Part print with two shaded views. Sizes in mm from the minimum x, y, z corner. A direction names the side the tool comes from. Give positions to 0.01 mm unless a question says otherwise; leave off trailing zeros. Order: outer loops, then holes, each group sorted by start corner. A loop starts at its lowest first (then second) coordinate and runs counter-clockwise, first axis right, second up. Notation, with made-up numbers: (-2.5, 0.25) -> (17.5, 0.25) arc R8 cw to (17.5, 12.25) -> close; hole circle Ø10 at (46, 16). An arc over 180 degrees is marked (long way). Answer as CSV lines item,"result".
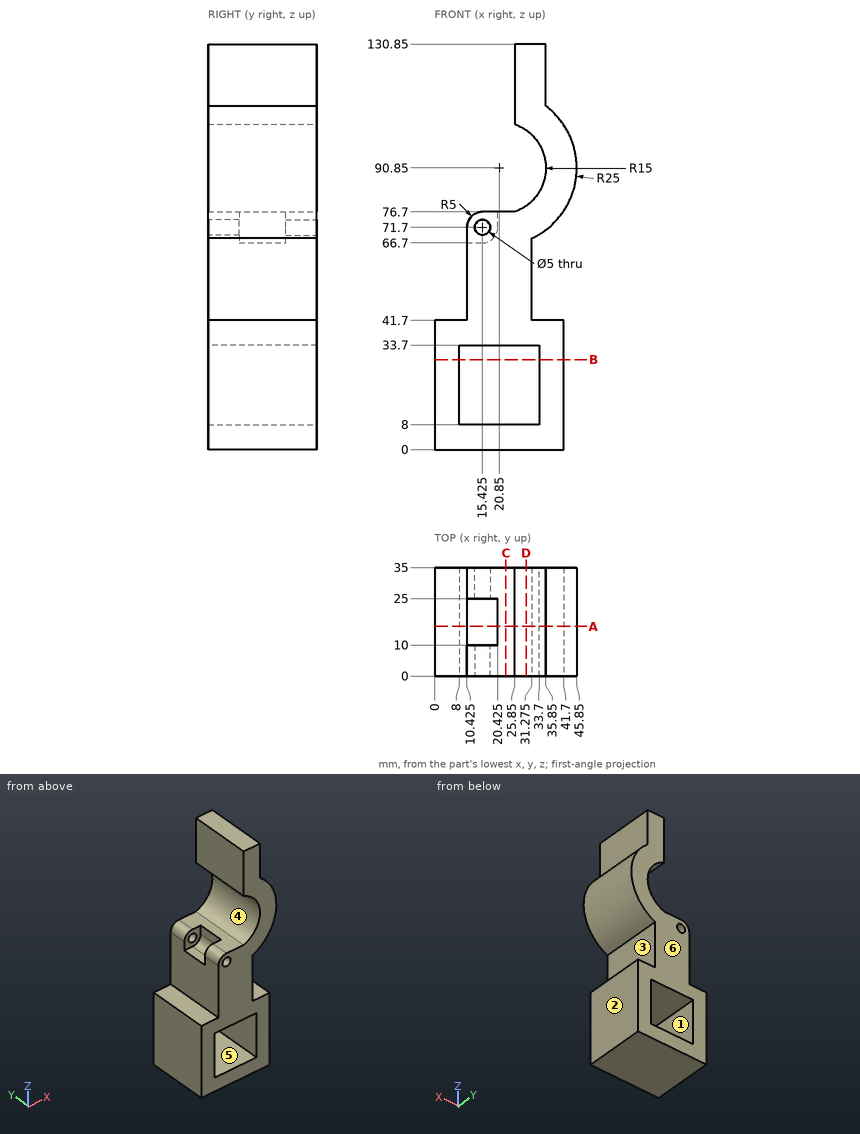
1) Band-saw the part on D-D, the plane x = 29.5. Write the cut outline in (y, z), then the cut area to 3 significant figures.
Data:
outline,"(0, 0) -> (35, 0) -> (35, 8) -> (0, 8) -> close; (0, 33.7) -> (35, 33.7) -> (35, 78.6) -> (0, 78.6) -> close; (0, 103.1) -> (35, 103.1) -> (35, 130.85) -> (0, 130.85) -> close"
area,"2,820 mm2"
2) Band-saw the part on A-A, the plane y = 16. Write the cut outline in (x, z) (3 decimals).
Data:
outline,"(0, 0) -> (41.7, 0) -> (41.7, 41.7) -> (31.275, 41.7) -> (31.275, 68.127) arc R25 ccw to (35.85, 110.85) -> (35.85, 130.85) -> (25.85, 130.85) -> (25.85, 104.992) arc R15 cw to (25.828, 76.7) -> (20.425, 76.7) -> (20.425, 71.7) arc R5 cw to (15.425, 66.7) -> (10.425, 66.7) -> (10.425, 41.7) -> (0, 41.7) -> close; hole (8, 8) -> (33.7, 8) -> (33.7, 33.7) -> (8, 33.7) -> close"
3) Band-saw the part on C-C, the plane x = 23. Write the cut outline in (y, z).
Data:
outline,"(0, 0) -> (35, 0) -> (35, 8) -> (0, 8) -> close; (0, 33.7) -> (35, 33.7) -> (35, 76.7) -> (0, 76.7) -> close"
4) Which spindle directions (+Z, -Z, +X, -X, +Y, -Y) get a long thin tool onto all of the face, cutting with end or side? Do the marked faces 1, 2 and 3. Say none if no direction does.
Data:
face 1,"+Y, -Y"
face 2,"-Z, +X, +Y, -Y"
face 3,"+X, +Y, -Y"
5) Wall check: line 1 along Z through (x, y) = (34.5, 34.5); line 2 along Z through (x, y) = (9, 24.5); line 3 along Z through (x, y) = (25, 4). Give the ranges that are in metal, low to high. Write a range as [from, to].
Data:
line 1,"z = [0, 41.7], [69.91, 84.63], [97.07, 130.85]"
line 2,"z = [0, 8], [33.7, 41.7]"
line 3,"z = [0, 8], [33.7, 76.7]"
6) Pull direction X, two halves, no side cores. Call the marked faces 4, 5 and 6: pulls with the +X half, pulls with the -X half, needs draft (parallel to the pull), parting line crosses it, or undercut.
Data:
face 4,"pulls with the -X half"
face 5,"undercut"
face 6,"needs draft"
7) Pin check, flat tips, straight feed: P1, Ø12, axis at x = 22, z = 74, coming from the -Y side; P2, Ø12, axis at y = 11.5, z = 117.5, coming from the -X side; P3, Ø3, axis at y = 26, z = 76.5, coming from the -X side; P4, Ø10, axis at y = 19, z = 27, coming from the +X side. Stop position of each tip, or through.
Data:
P1,"stops at y = 0"
P2,"stops at x = 25.85"
P3,"stops at x = 11.67"
P4,"stops at x = 41.7"
8) Band-saw the part on B-B, the plane z = 29. Write the cut outline in (x, y).
Data:
outline,"(0, 0) -> (8, 0) -> (8, 35) -> (0, 35) -> close; (33.7, 0) -> (41.7, 0) -> (41.7, 35) -> (33.7, 35) -> close"
